Geometry check sheet. Reference: the model listing, model coordinates, mm. A direction names the side the tool comes from. Round coordinates to 2 decimals unless told otherwise and drop trailing zeros. Order: outer loops, then holes, each group sorted by start corner. A loop starts at its lowest first (then second) coordinate and runs counter-clockwise, first axis right, second up. Notation, with made-up numbers: (-30, 71.5) - (-15, 71.5) arc R22 cw to (-15, 105.5) - close; hole circle Ø2 at (-34.5, 59). An arc over 180 degrees is marked (long way). Return JSON: item names as keys, results as strings. Group by question number.
Q1. Gauge pin test, flat ends, axial feed: pin 1 Ø1.5 at (x, y) = (0, 1.5) entering from +Z; pin 2 Ø1.6 at (x, z) = (33.5, 0) entering from -Y; pin 3 Ø0.6 at (x, y) = (-4.5, 1) entering from +Z. Record the tip position at first contact, or that the pin passes through.
Q2. Draft check along X on faces 1 (the cylindrical face through (-0.96, 0.49, 2.31)), 2 (the flat face through (10, 0, 0)). Enter one of: pulls with the +X half, pulls with the -X half, needs draft (parallel to the pull), parting line crosses it, or undercut.
Q3. Sectioned sample at A-A, the plane y = 1.5. Record the cut outline in (x, z).
Q4. Tool access check on faces 3 (the cylindrical face through (-2, 2, 0)), 4 (the cylindrical face through (30.751, 0.493, 2.385)), 5 (the flat face through (30, 0, 0)). Record the directions out of +Z, -Z, +X, -X, +Y, -Y that give a thin tool (end or side, any length) a straight path to the whole face; none if there is none.
Q5. Material ranges on line 1 along X through (y, z) = (2.3, 0.1); line 2 along X through (y, z) = (0.3, 0.2); line 3 along Y through (x, z) = (16.5, -0.5), recorded low to high.
Q6. Sectioned sample at B-B, the plane x = 23.5. Record the cut outline in (y, z).
```python
from build123d import *

# Parameters (mm, degrees)
SKETCH1_R           = 2
BOSS_EXTRUDE1_DEPTH = 3
SKETCH3_R           = 2.5
BOSS_EXTRUDE3_DEPTH = 1
LPATTERN4_COUNT     = 4
LPATTERN4_PITCH     = 10
SKETCH4_W           = 45
SKETCH4_H           = 2
BOSS_EXTRUDE4_DEPTH = 0.5


with BuildPart() as part:
    # Sketch1 → Boss-Extrude1 (new body)
    with BuildSketch(Plane(origin=(0, 0, 0), x_dir=(1, 0, 0), z_dir=(0, 1, 0))):
        with Locations(Location((0, 0, 0), (0, 0, 270))):
            Circle(SKETCH1_R)
    extrude(amount=BOSS_EXTRUDE1_DEPTH)

    # Sketch2 → Cut-Revolve1 (revolve, cut)
    with BuildSketch(Plane(origin=(0, 0, 0), x_dir=(0, 0, -1), z_dir=(1, 0, 0))):
        Polygon((0, 3), (0, 2.6), (-2, 3), align=None)
    revolve(axis=Axis((0, 3, 0), (0, -1, 0)), mode=Mode.SUBTRACT)

    # Sketch3 → Boss-Extrude3 (add)
    with BuildSketch(Plane(origin=(0, 0, 0), x_dir=(1, 0, 0), z_dir=(0, 1, 0))):
        with Locations(Location((0, 0, 0), (0, 0, 270))):
            Circle(SKETCH3_R)
    extrude(amount=BOSS_EXTRUDE3_DEPTH)


with BuildPart() as lpattern4_1:
    # LPattern4: pattern copy
    add(part.part.moved(Location(Vector(1, 0, 0) * (1 * LPATTERN4_PITCH))))


with BuildPart() as lpattern4_2:
    # LPattern4: pattern copy
    add(part.part.moved(Location(Vector(1, 0, 0) * (2 * LPATTERN4_PITCH))))


with BuildPart() as lpattern4_3:
    # LPattern4: pattern copy
    add(part.part.moved(Location(Vector(1, 0, 0) * (3 * LPATTERN4_PITCH))))


with BuildPart() as part_1:
    add(part.part)

    add(lpattern4_1.part)  # Boss-Extrude4 merges LPattern4_1

    add(lpattern4_2.part)  # Boss-Extrude4 merges LPattern4_2

    add(lpattern4_3.part)  # Boss-Extrude4 merges LPattern4_3
    # Sketch4 → Boss-Extrude4 (add)
    with BuildSketch(Plane(origin=(0, 1, 0), x_dir=(1, 0, 0), z_dir=(0, 1, 0))):
        with Locations((15, 0)):
            Rectangle(SKETCH4_W, SKETCH4_H)
    extrude(amount=-BOSS_EXTRUDE4_DEPTH)


solid = part_1.part
```
Reply:
{
 "1": {"pin 1": "z = 2.5", "pin 2": "y = 0.5", "pin 3": "z = 1"},
 "2": {"face 1": "undercut", "face 2": "needs draft"},
 "3": {"outline": "circle Ø4 at (0, 0); circle Ø4 at (10, 0); circle Ø4 at (20, 0); circle Ø4 at (30, 0)"},
 "4": {"face 3": "+Y", "face 4": "-Y", "face 5": "+Z, -Z, +X, -X, -Y"},
 "5": {"line 1": "-2 to 2, 8 to 12, 18 to 22, 28 to 32", "line 2": "-2.49 to 2.49, 7.51 to 12.49, 17.51 to 22.49, 27.51 to 32.49", "line 3": "0.5 to 1"},
 "6": {"outline": "(0.5, -1) - (1, -1) - (1, 1) - (0.5, 1) - close"}
}
